Design review of the part built by this model. Coordinates are the model's own, in mm. Face numbers are marked on the shaded views. A direction names the side the tool comes from. Coordinates: 2 decimals unless noted, no trailing zeros. Loops run counter-clockwise (first coordinate to the right, second up) from the corner with the lowest first, then second, coordinate; pieces in that order, holes last. Notation, with made-up numbers: (-31.5, -22) - (-2.5, -22) arc R29 ccw to (-2.5, 16) - close; hole circle Ø5 at (59.25, -33). An arc over 180 degrees is marked (long way). Answer in a Markdown table with one row per item. Add a question column.
(1) We need section A-A, the plane y = 0. Write out the cut boundary in (x, z).
(2) The part is to be moulded in two halves that separate along Y. For the marked faces 3, 4 and 5, say which applies: released by +Y, released by -Y, zero draft, split by the parting line, or undercut.
(3) To check wall thickness, follow L1, parallel to Y at x = 0, z = 4.75; L2, parallel to Y at x = 0, z = 15.6; L3, parallel to Z at x = -1.25, y = 1.5. State the ranges of each line that lie inside material, in increasing order. Write a range as [from, to].
(4) For the marked faces 1 and 2, list the 3-axis set-ups (+Z, -Z, +X, -X, +Y, -Y) from which the entire face can be reached by the end or side of a thin tool; tool diameter is ignored.
(5) We need section B-B, the plane z = 8. Write out the cut boundary in (x, y), plus the area to 3 significant figures.
(6) Clearance check with flat-ended pins moving along their axes: pin 1 (2.5 mm diameter, centred on x = 0, y = 0, fed in from -Z); pin 2 (1.5 mm diameter, centred on y = 2.5, z = 16, fed in from -X); pin 3 (1 mm diameter, centred on y = 3.5, z = 5.5, fed in from -X); pin 4 (1 mm diameter, centred on x = 2, z = 5.5, fed in from +Y). State where each tip first meets the part, or that it passes through.
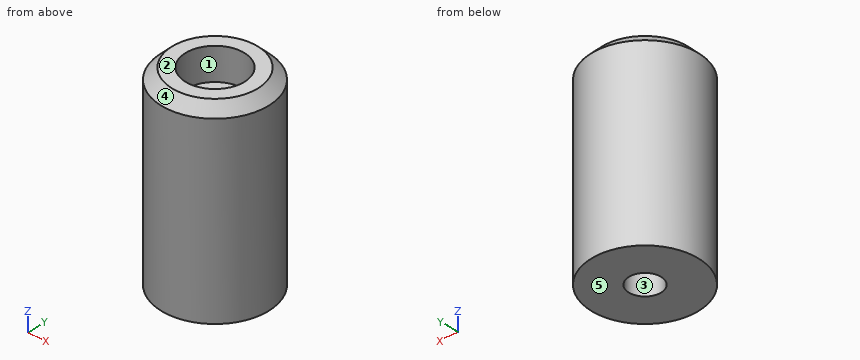
from build123d import *

# Parameters (mm, degrees)
SKETCH_R     = 5
SKETCH_R_2   = 1.5
PAD_DEPTH    = 18
SKETCH001_R  = 2.75
POCKET_DEPTH = 3
CHAMFER_SIZE = 1


with BuildPart() as part:
    # Sketch → Pad (new body)
    with BuildSketch(Plane.XY):
        Circle(SKETCH_R)
        Circle(SKETCH_R_2, mode=Mode.SUBTRACT)
    extrude(amount=PAD_DEPTH)

    # Sketch001 (on Face4 of Pad) → Pocket (cut)
    with BuildSketch(Plane.XY.offset(18)):
        Circle(SKETCH001_R)
    extrude(amount=-POCKET_DEPTH, mode=Mode.SUBTRACT)

    # Chamfer
    chamfer_edges = [part.edges().sort_by_distance(p)[0] for p in [
        (-5, 0, 18),
    ]]
    chamfer(chamfer_edges, length=CHAMFER_SIZE)


solid = part.part
Responses:
| question | item | result |
|---|---|---|
| 1 | outline | (-5, 0) - (-1.5, 0) - (-1.5, 15) - (-2.75, 15) - (-2.75, 18) - (-4, 18) - (-5, 17) - close; (1.5, 0) - (5, 0) - (5, 17) - (4, 18) - (2.75, 18) - (2.75, 15) - (1.5, 15) - close |
| 2 | face 3 | undercut |
| 2 | face 4 | split by the parting line |
| 2 | face 5 | zero draft |
| 3 | L1 | y = [-5, -1.5], [1.5, 5] |
| 3 | L2 | y = [-5, -2.75], [2.75, 5] |
| 3 | L3 | z = [0, 15] |
| 4 | face 1 | +Z |
| 4 | face 2 | +Z, +X, -X, +Y, -Y |
| 5 | outline | circle Ø10 at (0, 0); hole circle Ø3 at (0, 0) |
| 5 | area | 71.5 mm2 |
| 6 | pin 1 | passes through |
| 6 | pin 2 | stops at x = -4.68 |
| 6 | pin 3 | stops at x = -4 |
| 6 | pin 4 | stops at y = 4.77 |
